For this review, take the finished solid that the model builds, in its own axes (mm). Give positions to 0.01 mm unless a question says otherwise; leave off trailing zeros. Order: outer loops, then holes, each group sorted by start corner. A loop starts at its lowest first (then second) coordinate and runs counter-clockwise, first axis right, second up. Notation, with made-up numbers: (19, 62) - (69, 62) arc R19 cw to (69, 90) - close; hole circle Ø2 at (-0.75, 25). An arc over 180 degrees is marked (long way). Use a Markdown table: item, result. Add a question column.
1) Wall thickness on L1, parallel to Z at x = -33.5, y = 2; L2, parallel to X at y = 1.4, z = 9; L3, parallel to X at y = 2, z = 13: over which ranges is each line inside the solid? List them lowest first.
2) Clearance check with a flat-ended pin moving along its axis: P1, Ø2, axis at y = 1.5, z = 43, coming from the -X side. State where the tip first meets the part, or that it passes through.
3) We need section A-A on z = 43. Write out the cut boundary in (x, y).
```python
from build123d import *

# Parameters (mm, degrees)
BOSS_EXTRUDE1_DEPTH = 50.8
FILLET1_R           = 3.175


with BuildPart() as part:
    # Sketch1 → Boss-Extrude1 (new body)
    with BuildSketch(Plane.XY):
        Polygon((-38.1, 2.38125), (38.1, 2.38125), (33.3375, -2.38125), (-33.3375, -2.38125), align=None)
    extrude(amount=BOSS_EXTRUDE1_DEPTH)

    # Fillet1
    fillet1_edges = [part.edges().sort_by_distance(p)[0] for p in [
        (35.71875, 0, 50.8),
        (-35.71875, 0, 50.8),
        (35.71875, 0, 0),
        (-35.71875, 0, 0),
    ]]
    fillet(fillet1_edges, radius=FILLET1_R)


solid = part.part
```
Checked values:
| question | item | result |
|---|---|---|
| 1 | L1 | 0.01 to 50.79 |
| 1 | L2 | -37.12 to 37.12 |
| 1 | L3 | -37.72 to 37.72 |
| 2 | P1 | x = -38.1 |
| 3 | outline | (-38.1, 2.38) - (-33.34, -2.38) - (33.34, -2.38) - (38.1, 2.38) - close |
